Check sheet for the modelled part. Datum: model origin and axes. Units: mm. A direction names the side the tool comes from. Round coordinates to 2 decimals unless told otherwise and drop trailing zeros. Write each loop counter-clockwise with the first axis right and the second up, starting at its lowest first coordinate (ties: lowest second). Pieces come first, ordered by that corner, then holes. Notation, with made-up numbers: M 17,73.5 L 41,73.5 A17 ccw 41,91.5 Z; hole C -20.75,-4 d7. An arc over 180 degrees is marked long. One line per item, written item: value.
from build123d import *

# Parameters (mm, degrees)
SKETCH1_W           = 15.6
SKETCH1_H           = 15.6
BOSS_EXTRUDE1_DEPTH = 10
SKETCH2_R           = 7.8
BOSS_EXTRUDE2_DEPTH = 16
SKETCH3_W           = 4
SKETCH3_H           = 4
CUT_EXTRUDE2_DEPTH  = 5.2


with BuildPart() as part:
    # Sketch1 → Boss-Extrude1 (new body)
    with BuildSketch(Plane(origin=(0, 0, 0), x_dir=(0, 0, -1), z_dir=(1, 0, 0))):
        Rectangle(SKETCH1_W, SKETCH1_H)
    extrude(amount=BOSS_EXTRUDE1_DEPTH)

    # Sketch2 → Boss-Extrude2 (add)
    with BuildSketch(Plane(origin=(10, 0, 0), x_dir=(0, 0, -1), z_dir=(1, 0, 0))):
        Circle(SKETCH2_R)
    extrude(amount=BOSS_EXTRUDE2_DEPTH)

    # Sketch3 → Cut-Extrude2 (cut)
    with BuildSketch(Plane(origin=(26, 0, 0), x_dir=(0, 0, -1), z_dir=(1, 0, 0))):
        with BuildLine():
            Line((-2, -2), (-2, 2))
            Line((-2, 2), (-7.53923073, 2))
            ThreePointArc((-7.53923073, 2), (-7.734532943, 1.008464255), (-7.8, 0))
            ThreePointArc((-7.8, 0), (-7.734532943, -1.008464255), (-7.53923073, -2))
            Line((-7.53923073, -2), (-2, -2))
        make_face()
        with BuildLine():
            ThreePointArc((2, 7.53923073), (1.008464255, 7.734532943), (0, 7.8))
            ThreePointArc((0, 7.8), (-1.008464255, 7.734532943), (-2, 7.53923073))
            Line((-2, 7.53923073), (-2, 2))
            Line((-2, 2), (2, 2))
            Line((2, 2), (2, 7.53923073))
        make_face()
        with BuildLine():
            Line((7.53923073, 2), (2, 2))
            Line((2, 2), (2, -2))
            Line((2, -2), (7.53923073, -2))
            ThreePointArc((7.53923073, -2), (7.734532943, -1.008464255), (7.8, 0))
            ThreePointArc((7.8, 0), (7.734532943, 1.008464255), (7.53923073, 2))
        make_face()
        with BuildLine():
            Line((2, -2), (-2, -2))
            Line((-2, -2), (-2, -7.53923073))
            ThreePointArc((-2, -7.53923073), (-1.008464255, -7.734532943), (0, -7.8))
            ThreePointArc((0, -7.8), (1.008464255, -7.734532943), (2, -7.53923073))
            Line((2, -7.53923073), (2, -2))
        make_face()
        with BuildLine():
            ThreePointArc((-7.53923073, -2), (-7.734532943, -1.008464255), (-7.8, 0))
            Line((-7.8, 0), (-7.8, -2))
            Line((-7.8, -2), (-7.53923073, -2))
        make_face()
        with BuildLine():
            ThreePointArc((-7.8, 0), (-7.734532943, 1.008464255), (-7.53923073, 2))
            Line((-7.53923073, 2), (-7.8, 2))
            Line((-7.8, 2), (-7.8, 0))
        make_face()
        with BuildLine():
            Line((0, 7.8), (-2, 7.8))
            Line((-2, 7.8), (-2, 7.53923073))
            ThreePointArc((-2, 7.53923073), (-1.008464255, 7.734532943), (0, 7.8))
        make_face()
        with BuildLine():
            Line((2, 7.8), (0, 7.8))
            ThreePointArc((0, 7.8), (1.008464255, 7.734532943), (2, 7.53923073))
            Line((2, 7.53923073), (2, 7.8))
        make_face()
        with BuildLine():
            Line((7.8, 2), (7.53923073, 2))
            ThreePointArc((7.53923073, 2), (7.734532943, 1.008464255), (7.8, 0))
            Line((7.8, 0), (7.8, 2))
        make_face()
        with BuildLine():
            Line((7.8, -2), (7.8, 0))
            ThreePointArc((7.8, 0), (7.734532943, -1.008464255), (7.53923073, -2))
            Line((7.53923073, -2), (7.8, -2))
        make_face()
        Rectangle(SKETCH3_W, SKETCH3_H)
    extrude(amount=-CUT_EXTRUDE2_DEPTH, mode=Mode.SUBTRACT)


solid = part.part
Q1. Depth check by flat-ended pin: P1, Ø4, axis at x = 24, z = -3.5, coming from the +Y side; P2, Ø1.6, axis at x = 23, z = -5, coming from the -Y side; P3, Ø5.5, axis at x = 22.5, z = 5, coming from the -Y side. Enter the tip coordinate at first touch or a pass-through.
Completed:
P1: y = 7.54
P2: y = -6.57
P3: y = -7.47
Q2. Sectioned sample at B-B on z = -5.5. Enter the section's corners in (x, y), and give its area (3 significant figures).
Completed:
outline: M 0,-7.8 L 10,-7.8 L 10,-5.53 L 26,-5.53 L 26,-2 L 20.8,-2 L 20.8,2 L 26,2 L 26,5.53 L 10,5.53 L 10,7.8 L 0,7.8 Z
area: 312 mm^2
Q3. Scan lines: line 1 (Y direction, x = 22.25, z = 3.5); line 2 (Z direction, x = 16.5, y = -2); line 3 (X direction, y = 7.25, z = 7). Record each from-to range of solid material in increasing order. Write a range as [from, to].
Completed:
line 1: [-6.97, -2], [2, 6.97]
line 2: [-7.54, 7.54]
line 3: [0, 10]
Q4. Access from +Z, -Z, +X, -X, +Y, -Y to the whole of each face (thin tool, end or side, straight path). Record for faces 4 (the flat face through (23, 2, 5)), 5 (the flat face through (10, 6, 6)), 6 (the flat face through (10, 6, -6)), 7 (the flat face through (23, -5, -2)).
Completed:
face 4: +Z, -Z, +X
face 5: +Z, +X, +Y
face 6: -Z, +X, +Y
face 7: +X, +Y, -Y
Q5. Draft check along Z on faces 1 (the flat face through (23, 5, -2)), 2 (the flat face through (0, 0, 0)), 3 (the cylindrical face through (17.89, 2.34, -7.44)). Enter one of: pulls with the +Z half, pulls with the -Z half, needs draft (parallel to the pull), parting line crosses it, or undercut.
Completed:
face 1: undercut
face 2: needs draft
face 3: parting line crosses it
Q6. Sectioned sample at A-A on x = 21.5. Enter the section's corners in (y, z).
Completed:
outline: M -7.54,-2 A7.8 ccw -2,-7.54 L -2,-2 Z; M -7.54,2 L -2,2 L -2,7.54 A7.8 ccw Z; M 2,-7.54 A7.8 ccw 7.54,-2 L 2,-2 Z; M 2,2 L 7.54,2 A7.8 ccw 2,7.54 Z
